Geometry: see drawing. Coordinates: mm, zero at the bounding-box minimum. A direction names the side the tool comes from. Coordinates: 2 decimals unless noted, no trailing zeros. Order: outer loops, then holes, each group sorted by start corner. A loop starts at its lowest first (then second) coordinate and runs counter-clockwise, first axis right, second up.
Item 1: Section C-C on x = 4. Return the cut outline in (y, z).
Item 2: Contact query for flat-ended pins moving along their axis: P1, Ø1.1, axis at x = 3.5, z = 3.5, coming from the +Y side; P2, Ø1.5, axis at y = 11, z = 2, coming from the +X side; P3, Ø3, axis at x = 4, y = 2.5, coming from the -Z side; P4, Ø1.5, axis at x = 2, y = 13.5, coming from the -Z side. Output: stop coordinate, or through.
Item 3: Ray query, line 1 (Y direction, x = 4, z = 3.85); line 2 (Z direction, x = 6.5, y = 1.25); line 3 (X direction, y = 6, z = 2). Return the intervals inside material, ascending.
Item 4: Section A-A on y = 2.5. Return the cut outline in (x, z).
Item 5: Mould query, pull axis Y, two halves, no side actions, for the marked faces 1, 2 and 3. Classes: released by +Y, released by -Y, zero draft, split by the parting line, or undercut.
Item 6: Section B-B on z = 3.7. Return the cut outline in (x, y).
Item 7: Section D-D on y = 1. Return the cut outline in (x, z).
Item 8: Reachability of the marked faces 4, 5 and 6 from +Z, -Z, +X, -X, +Y, -Y: full face, straight path, thin tool, end or side. Return the list, or none.
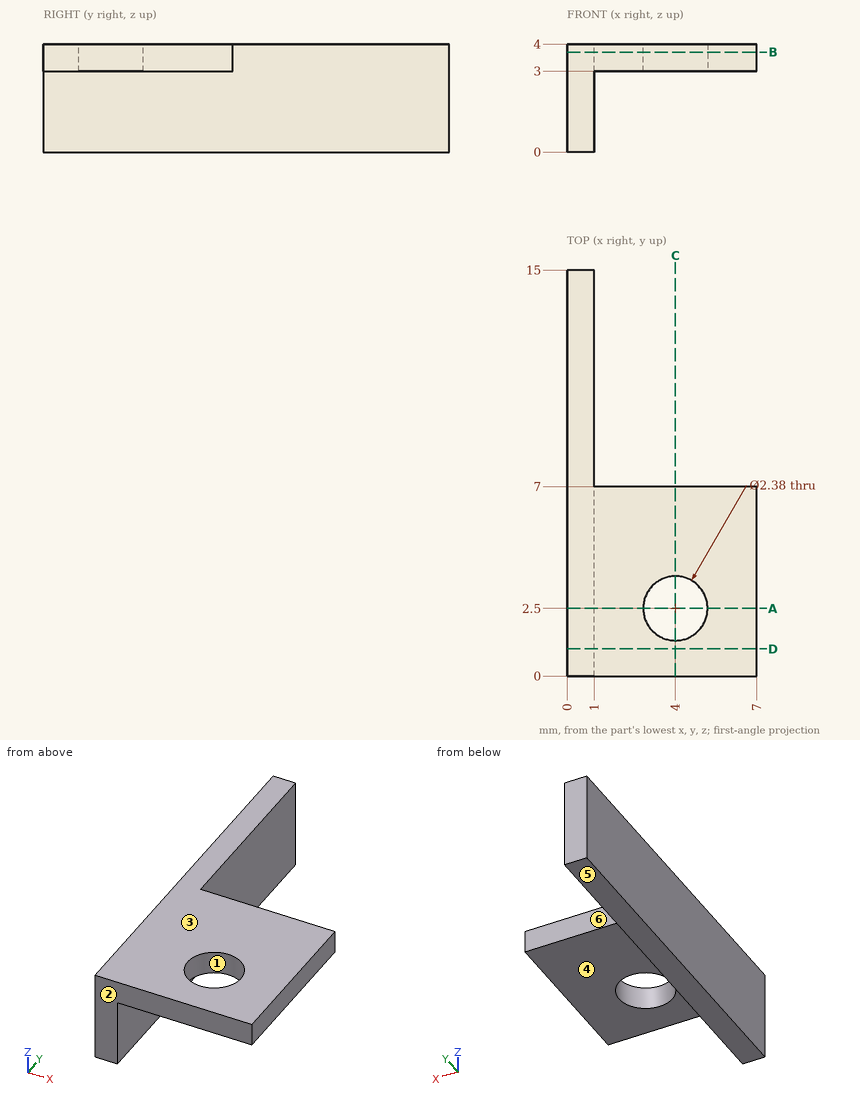
Answer list:
1. outline: (0, 3) - (1.31, 3) - (1.31, 4) - (0, 4) - close; (3.69, 3) - (7, 3) - (7, 4) - (3.69, 4) - close
2. P1: stops at y = 7
2. P2: stops at x = 1
2. P3: stops at z = 3
2. P4: passes through
3. line 1: y = 0 to 1.31, 3.69 to 7
3. line 2: z = 3 to 4
3. line 3: x = 0 to 1
4. outline: (0, 0) - (1, 0) - (1, 3) - (2.81, 3) - (2.81, 4) - (0, 4) - close; (5.19, 3) - (7, 3) - (7, 4) - (5.19, 4) - close
5. face 1: undercut
5. face 2: released by -Y
5. face 3: zero draft
6. outline: (0, 0) - (7, 0) - (7, 7) - (1, 7) - (1, 15) - (0, 15) - close; hole circle Ø2.38 at (4, 2.5)
7. outline: (0, 0) - (1, 0) - (1, 3) - (7, 3) - (7, 4) - (0, 4) - close
8. face 4: -Z, +X, +Y, -Y
8. face 5: -Z, +X, -X, +Y, -Y
8. face 6: +Z, -Z, +X, +Y
